For this review, use the dimensioned drawing (mm, ordinates from the lowest corner) and the shaded views. Give positions to 0.01 mm unless a question says otherwise; leave off trailing zeros. Write each loop counter-clockwise with the first axis right and the second up, starting at its lowest first coordinate (ties: lowest second). Pieces come first, ordered by that corner, then holes. Notation, with made-up numbers: (-22.5, 26.5) - (15.5, 26.5) arc R27 cw to (15.5, 62.5) - close; hole circle Ø5 at (-36, 50.25). An arc over 180 degrees is marked (long way). One line per question, with ' | ' between items. Start each with the question number.
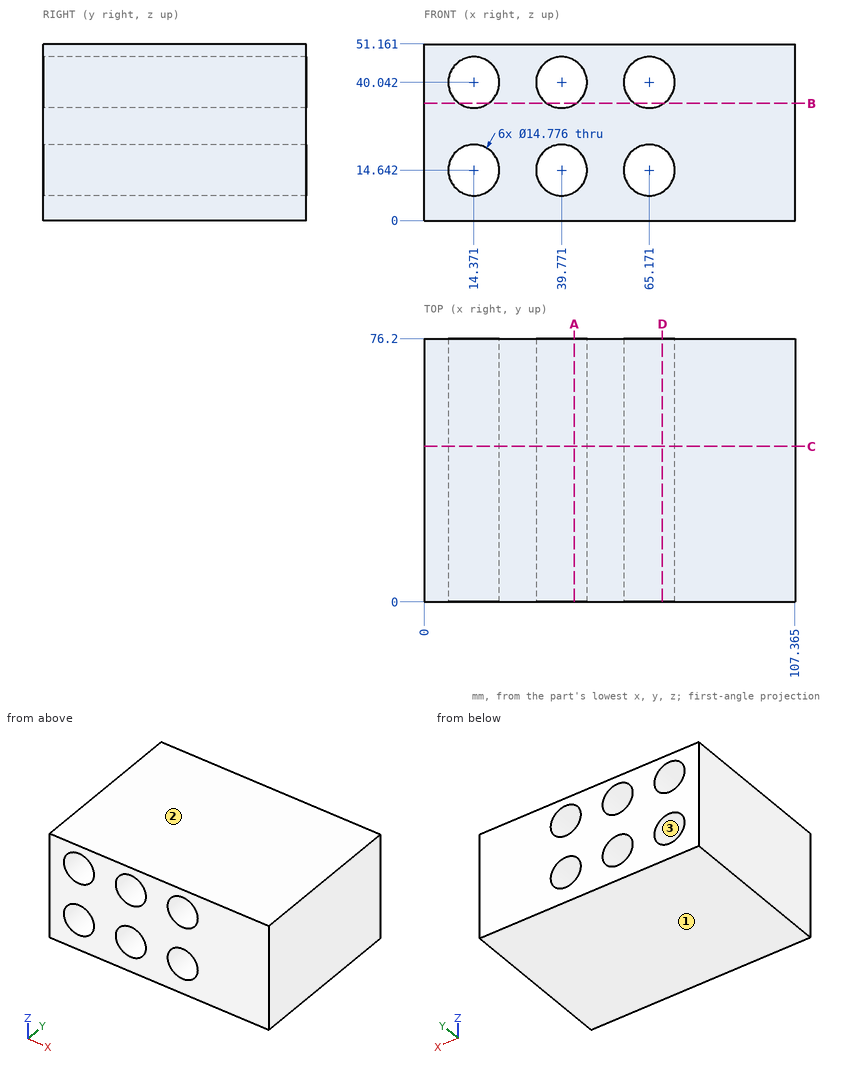
Item 1: Take a section at D-D (x = 69). Give the boundary of the cut face in (y, z), plus the area to 3 significant figures.
Item 2: Take a section at B-B (z = 34). Give the boundary of the cut face in (x, y) (1 decimal), plus the area to 3 significant figures.
Item 3: Take a section at A-A (x = 43.5). Give the boundary of the cut face in (y, z).
Item 4: Take a section at C-C (y = 45). Give the boundary of the cut face in (x, z) (1 decimal).
Item 5: Clearance check with a flat-ended pin moving along its axis: P1, Ø8, axis at x = 56.5, z = 37.5, coming from the -Y side. State where the tip first meets the part, or that it passes through.
Item 6: The part is to be moulded in two halves that separate along Z. For the marked faces 1, 2 and 3, say which applies: +Z half, -Z half, draft (parallel to the pull), parting line (faces both ways), or undercut.
Item 7: For probe 1 along X at (y, z) = (71.5, 14.5) (1 decimal); probe 2 along X at (y, z) = (43, 35) (1 decimal); probe 3 along Z at (x, y) = (60, 39.5) (1 decimal), list the stretches that pass through material, from the lowest coordinate up.
Check sheet entries:
1) outline: (0, 0) - (76.2, 0) - (76.2, 8.32) - (0, 8.32) - close; (0, 20.96) - (76.2, 20.96) - (76.2, 33.72) - (0, 33.72) - close; (0, 46.36) - (76.2, 46.36) - (76.2, 51.16) - (0, 51.16) - close | area: 1,970 mm^2
2) outline: (0, 0) - (10.1, 0) - (10.1, 76.2) - (0, 76.2) - close; (18.6, 0) - (35.5, 0) - (35.5, 76.2) - (18.6, 76.2) - close; (44, 0) - (60.9, 0) - (60.9, 76.2) - (44, 76.2) - close; (69.4, 0) - (107.4, 0) - (107.4, 76.2) - (69.4, 76.2) - close | area: 6,240 mm^2
3) outline: (0, 0) - (76.2, 0) - (76.2, 8.26) - (0, 8.26) - close; (0, 21.02) - (76.2, 21.02) - (76.2, 33.66) - (0, 33.66) - close; (0, 46.42) - (76.2, 46.42) - (76.2, 51.16) - (0, 51.16) - close
4) outline: (0, 0) - (107.4, 0) - (107.4, 51.2) - (0, 51.2) - close; hole circle Ø14.8 at (14.4, 14.6); hole circle Ø14.8 at (14.4, 40); hole circle Ø14.8 at (39.8, 14.6); hole circle Ø14.8 at (39.8, 40); hole circle Ø14.8 at (65.2, 14.6); hole circle Ø14.8 at (65.2, 40)
5) P1: stops at y = 0
6) face 1: -Z half | face 2: +Z half | face 3: undercut
7) probe 1: x = 0 to 7, 21.8 to 32.4, 47.2 to 57.8, 72.6 to 107.4 | probe 2: x = 0 to 9, 19.8 to 34.4, 45.2 to 59.8, 70.6 to 107.4 | probe 3: z = 0 to 9.4, 19.9 to 34.8, 45.3 to 51.2
